Here's how the part is built. I have some questions about the finished solid (model axes, mm). Face numbers are marked on the shaded views. Round coordinates to 2 decimals unless told otherwise and drop trailing zeros. Write each loop counter-clockwise with the first axis right and the second up, starting at its lowest first coordinate (ties: lowest second). Pieces come first, ordered by that corner, then holes. Notation, with made-up numbers: (42.5, 54.5) -> (54.5, 54.5) arc R17 ccw to (54.5, 71.5) -> close; hole circle Ø11 at (12.25, 14). An arc over 180 degrees is marked (long way). Answer in a Markdown table with one row per item.
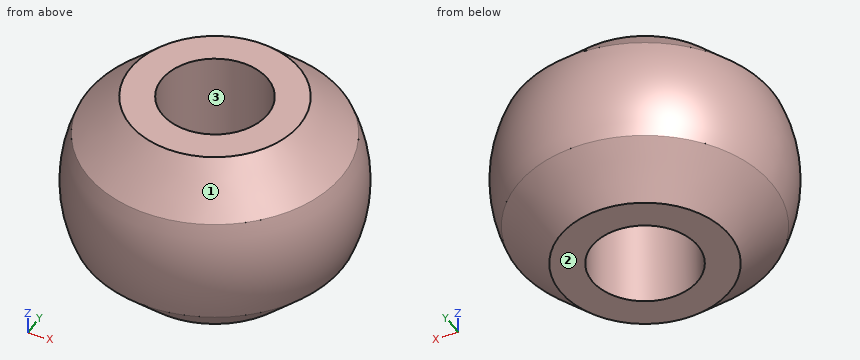
from build123d import *

# Parameters (mm, degrees)
SKETCH_1_R          = 10
EXTRUDE_1_DEPTH     = 4.5
SKETCH_4_R          = 8
EXTRUDE_3_DEPTH     = 5
SKETCH_5_R          = 8
EXTRUDE_4_DEPTH     = 2.5
SKETCH_8_R          = 4
SKETCH_7_R          = 6
SKETCH_9_R          = 14.627232323
SKETCH_9_R_2        = 10
CUT_EXTRUDE_1_DEPTH = 18
SKETCH_10_R         = 2.5
CUT_EXTRUDE_2_DEPTH = 10
SKETCH_2_R          = 6
EXTRUDE_5_DEPTH     = 80
SKETCH_11_W         = 44.642823809
SKETCH_11_H         = 125.571137761
SKETCH_11_R         = 6
CUT_EXTRUDE_3_DEPTH = 18


with BuildPart() as part:
    # 草图1 → 凸台-拉伸1 (new body)
    with BuildSketch(Plane(origin=(0, 0, 0), x_dir=(1, 0, 0), z_dir=(0, 1, 0))):
        with Locations(Location((0, 0, 0), (0, 0, 270))):
            Circle(SKETCH_1_R)
    extrude(amount=EXTRUDE_1_DEPTH)

    # 草图4 → 凸台-拉伸3 (add, symmetric)
    with BuildSketch(Plane.XY):
        with BuildLine():
            Line((-10, 4.5), (10, 4.5))
            Line((10, 4.5), (10, 14.5))
            ThreePointArc((10, 14.5), (0, 24.5), (-10, 14.5))
            Line((-10, 14.5), (-10, 4.5))
        make_face()
        with Locations((0, 14.5)):
            Circle(SKETCH_4_R, mode=Mode.SUBTRACT)
    extrude(amount=EXTRUDE_3_DEPTH, both=True)

    # 草图5 → 凸台-拉伸4 (add, symmetric)
    with BuildSketch(Plane.XY):
        with Locations((0, 14.5)):
            Circle(SKETCH_5_R)
    extrude(amount=EXTRUDE_4_DEPTH, both=True)

    # 草图8 → 放样1 section 0
    with BuildSketch(Plane.XY.offset(4.5)):
        with Locations((0, 14.5)):
            Circle(SKETCH_8_R)
    # 草图7 → 放样1 section 1
    with BuildSketch(Plane.XY.offset(2.5)):
        with Locations((0, 14.5)):
            Circle(SKETCH_7_R)
    loft_1 = loft()

    # 镜向1: 放样1 across plane
    add(loft_1.mirror(Plane.XY))

    # 草图9 → 切除-拉伸1 (cut)
    with BuildSketch(Plane(origin=(0, 4.5, 0), x_dir=(1, 0, 0), z_dir=(0, 1, 0))):
        Circle(SKETCH_9_R)
        with Locations(Location((0, 0, 0), (0, 0, 150))):
            Circle(SKETCH_9_R_2, mode=Mode.SUBTRACT)
    extrude(amount=CUT_EXTRUDE_1_DEPTH, mode=Mode.SUBTRACT)

    # 草图10 → 切除-拉伸2 (cut)
    with BuildSketch(Plane.XY.offset(4.5)):
        with Locations((0, 14.5)):
            Circle(SKETCH_10_R)
    extrude(amount=-CUT_EXTRUDE_2_DEPTH, mode=Mode.SUBTRACT)

    # 草图2 → 凸台-拉伸5 (add)
    with BuildSketch(Plane.XZ):
        with Locations(Location((0, 0, 0), (0, 0, 270))):
            Circle(SKETCH_2_R)
    extrude(amount=EXTRUDE_5_DEPTH)

    # 草图11 → 切除-拉伸3 (cut, symmetric)
    with BuildSketch(Plane.XY.offset(4.5)):
        with Locations((1.10319776, -29.667351992)):
            Rectangle(SKETCH_11_W, SKETCH_11_H)
        with Locations(Location((0, 14.5, 0), (0, 0, 180))):
            Circle(SKETCH_11_R, mode=Mode.SUBTRACT)
    extrude(amount=CUT_EXTRUDE_3_DEPTH, both=True, mode=Mode.SUBTRACT)

    # 草图13 → 旋转2 (revolve)
    with BuildSketch(Plane(origin=(0, 0, 0), x_dir=(0, 0, -1), z_dir=(1, 0, 0)), mode=Mode.PRIVATE) as revolve_2_sk:
        with BuildLine():
            Line((-2.5, 20.5), (2.5, 20.5))
            ThreePointArc((2.5, 20.5), (0, 21), (-2.5, 20.5))
        make_face()
    revolve(revolve_2_sk.sketch.rotate(Axis((0, 14.5, 0), (0, 0, -1)), 270), axis=Axis((0, 14.5, 0), (0, 0, -1)))


solid = part.part
1) I want a section at C-C, the plane z = 1.5. List the corners of the cut face in (x, y) for me, and give its area (3 significant figures).
Response:
| item | result |
|---|---|
| outline | circle Ø12.65 at (0, 14.5); hole circle Ø5 at (0, 14.5) |
| area | 106 mm^2 |
2) We'd pull the mould along X, two halves only. Please class the marked faces 1, 2 and 3: +X half, -X half, draft (parallel to the pull), parting line (faces both ways), or undercut.
Response:
| item | result |
|---|---|
| face 1 | parting line |
| face 2 | draft |
| face 3 | undercut |
3) I need wall thicknesses on line 1 (Y direction, x = 0, z = 0.5); line 2 (Y direction, x = 0, z = -2); line 3 (Z direction, x = 3.5, y = 9.5). Which ranges of each line are inside material? Lowest first, please. Write a range as [from, to].
Response:
| item | result |
|---|---|
| line 1 | y = [8.02, 12], [17, 20.98] |
| line 2 | y = [8.32, 12], [17, 20.68] |
| line 3 | z = [-2.24, 2.24] |
4) I want a section at B-B, the plane z = 3. List the corners of the cut face in (x, y) for me.
Response:
| item | result |
|---|---|
| outline | circle Ø11 at (0, 14.5); hole circle Ø5 at (0, 14.5) |
5) I want a section at A-A, the plane x = 0. List the corners of the cut face in (y, z) for me, and give its area (3 significant figures).
Response:
| item | result |
|---|---|
| outline | (8.5, -2.5) -> (10.5, -4.5) -> (12, -4.5) -> (12, 4.5) -> (10.5, 4.5) -> (8.5, 2.5) arc R6.5 ccw to start; (17, -4.5) -> (18.5, -4.5) -> (20.5, -2.5) arc R6.5 ccw to (20.5, 2.5) -> (18.5, 4.5) -> (17, 4.5) -> close |
| area | 58.4 mm^2 |
6) For pin 1 (5 mm diameter, centred on y = 19.5, z = 0, fed in from -X); pin 2 (3 mm diameter, centred on y = 10, z = -0.5, fed in from -X); pin 3 (1.5 mm diameter, centred on x = 5, z = -2.5, fed in from +Y), each with a flat end and sliding along its axis, tell me the tip position at first contact or that it passes through.
Response:
| item | result |
|---|---|
| pin 1 | stops at x = -6 |
| pin 2 | stops at x = -5.75 |
| pin 3 | stops at y = 18.84 |
